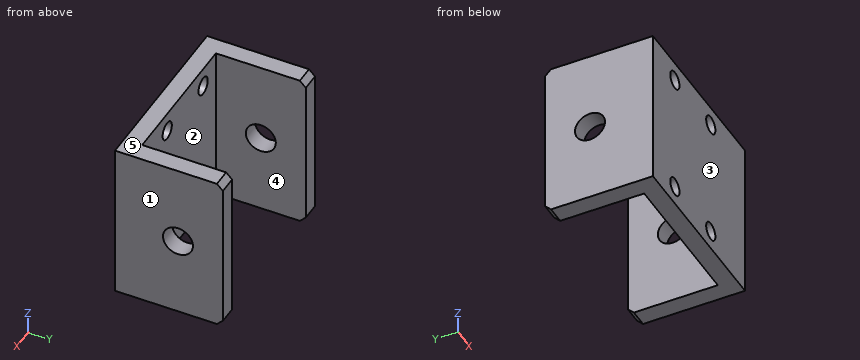
Autodesk Inventor part; units mm, degrees
ref_plane "YZ Plane" through (0, 0, 0) normal (1, 0, 0) x (0, 1, 0)
ref_plane "XZ Plane" through (0, 0, 0) normal (0, 1, 0) x (-1, 0, 0)
ref_plane "XY Plane" through (0, 0, 0) normal (0, 0, 1) x (1, 0, 0)
sketch "Szkic1" plane through (0, 0, 0) normal (0, 0, 1) x (1, 0, 0)
  line L0 (-6.4502, 4.7958) -> (-6.4502, -25.2042)
  line L1 (-6.4502, -25.2042) -> (23.5498, -25.2042)
  line L2 (23.5498, -25.2042) -> (23.5498, 4.7958)
  line L3 (-6.4502, 4.7958) -> (-3.4502, 4.7958)
  line L4 (-3.4502, 4.7958) -> (-3.4502, -22.2042)
  line L5 (23.5498, 4.7958) -> (20.5498, 4.7958)
  line L6 (20.5498, 4.7958) -> (20.5498, -22.2042)
  line L7 (20.5498, -22.2042) -> (-3.4502, -22.2042)
  point P0 (0, 0)
  dimension "d0" = 30
  dimension "d1" = 30
  dimension "d2" = 30
  dimension "d3" = 3
  dimension "d4" = 27
  dimension "d5" = 3
extrude "Wyciągnięcie proste1" add sketch "Szkic1" along normal blind 27
sketch "Szkic2" plane through (-6.4502, -25.2042, 0) normal (-1, 0, 0) x (0, 0, 1)
  line L0 (0, 30) -> (0, 0)
  line L1 (0, 0) -> (27, 0)
  line L2 (27, 30) -> (27, 0)
  line L3 (0, 30) -> (27, 30)
  line L4 (0, 3) -> (27, 3)
  circle A0 centre (13.5, 10.5) radius 2.5
  line L5 (27, 30) -> (27, 0)
  line L6 (27, 18) -> (0, 18)
  point P0 (0, 25.2042)
  dimension "d8" = 27
  dimension "d9" = 13.5
  dimension "d10" = 5
  dimension "d11" = 7.5
  dimension "d12" = 7.5
extrude "Wyciągnięcie proste2" cut sketch "Szkic2" against normal through all contours L3 L2 L6 L0 | A0
chamfer "Faza2" distance 1 angle 45 4 edges at (22.0498, -7.2042, 27) (-4.9502, -7.2042, 27) (22.0498, -7.2042, 0) (-4.9502, -7.2042, 0)
sketch "Szkic5" plane through (-6.4502, -25.2042, 0) normal (0, -1, 0) x (1, 0, 0)
  line L0 (0, 0) -> (30, 0)
  line L1 (30, 0) -> (30, 27)
  line L2 (0, 27) -> (30, 27)
  line L3 (0, 0) -> (0, 27)
  line L4 (3, 0) -> (3, 27)
  line L5 (27, 0) -> (27, 27)
  point P0 (6.4502, 0)
  point P1 (7.15, 23.75)
  point P2 (18.85, 23.75)
  point P3 (7.15, 3.25)
  point P4 (18.85, 3.25)
  dimension "d21" = 20.5
  dimension "d22" = 11.7
  dimension "d24" = 11.7
  dimension "d25" = 20.5
  dimension "d26" = 27
  dimension "d27" = 3.25
  dimension "d28" = 22.85
hole "Otwór1" at (0.6998, -25.2042, 23.75) at (12.3998, -25.2042, 23.75) at (0.6998, -25.2042, 3.25) at (12.3998, -25.2042, 3.25) direction (0, 1, 0) diameter 3 end through all
properties part number "CNCM_ALU_Y_Axis_Tensioning_System_C_Sec"
CAD build for the part. Positions are in the model's coordinates, mm. Face numbers are marked on the shaded views. A direction names the side the tool comes from. Round coordinates to 2 decimals unless told otherwise and drop trailing zeros. Order: outer loops, then holes, each group sorted by start corner. A loop starts at its lowest first (then second) coordinate and runs counter-clockwise, first axis right, second up.
Item 1: Mould opens along X. For the marked faces 1, 2 and 3 say: pulls with the +X half, pulls with the -X half, needs draft (parallel to the pull), parting line crosses it, or undercut.
Item 2: Pin check, flat tips, straight feed: pin 1 (5 mm diameter, centred on x = 12.4, z = 23.75, fed in from +Y); pin 2 (1.5 mm diameter, centred on x = 18, y = -16, fed in from -Z). Stop position of each tip, or through.
Item 3: Saw through at A-A on y = -20.5. Write the cut outline in (x, z), then the cut area to 3 significant figures.
Item 4: Saw through at B-B on z = 3.25. Write the cut outline in (x, y), then the cut area to 3 significant figures.
Item 5: Tool access for the marked faces 4 and 5: list every direction of +Z, -Z, +X, -X, +Y, -Y with a clear straight run to the whole face (end or side of a thin tool).
Item 6: Probe line 1 along X through (y, z) = (-24.3, 3.25); line 2 along Y through (x, z) = (21.25, 13.5); line 3 along X through (y, z) = (-18.75, 20.25). List the from-to ranges inside material, lowest first.
Item 7: Saw through at C-C on z = 8.5. Write the cut outline in (x, y).
Item 8: Saw through at D-D on z = 13.5. Write the cut outline in (x, y).
Reported:
1. face 1: pulls with the +X half
1. face 2: undercut
1. face 3: needs draft
2. pin 1: stops at y = -22.2
2. pin 2: passes through
3. outline: (-6.45, 0) - (-3.45, 0) - (-3.45, 27) - (-6.45, 27) - close; (20.55, 0) - (23.55, 0) - (23.55, 27) - (20.55, 27) - close
3. area: 162 mm2
4. outline: (-6.45, -25.2) - (-0.8, -25.2) - (-0.8, -22.2) - (-3.45, -22.2) - (-3.45, -7.2) - (-6.45, -7.2) - close; (2.2, -25.2) - (10.9, -25.2) - (10.9, -22.2) - (2.2, -22.2) - close; (13.9, -25.2) - (23.55, -25.2) - (23.55, -7.2) - (20.55, -7.2) - (20.55, -22.2) - (13.9, -22.2) - close
4. area: 162 mm2
5. face 4: +Z, -Z, +Y
5. face 5: +Z, +X, -X, +Y, -Y
6. line 1: x = -6.45 to -0.8, 2.2 to 10.9, 13.9 to 23.55
6. line 2: y = -25.2 to -17.2, -12.2 to -7.2
6. line 3: x = -6.45 to -3.45, 20.55 to 23.55
7. outline: (-6.45, -25.2) - (23.55, -25.2) - (23.55, -7.2) - (20.55, -7.2) - (20.55, -22.2) - (-3.45, -22.2) - (-3.45, -7.2) - (-6.45, -7.2) - close
8. outline: (-6.45, -25.2) - (23.55, -25.2) - (23.55, -17.2) - (20.55, -17.2) - (20.55, -22.2) - (-3.45, -22.2) - (-3.45, -17.2) - (-6.45, -17.2) - close; (-6.45, -12.2) - (-3.45, -12.2) - (-3.45, -7.2) - (-6.45, -7.2) - close; (20.55, -12.2) - (23.55, -12.2) - (23.55, -7.2) - (20.55, -7.2) - close
